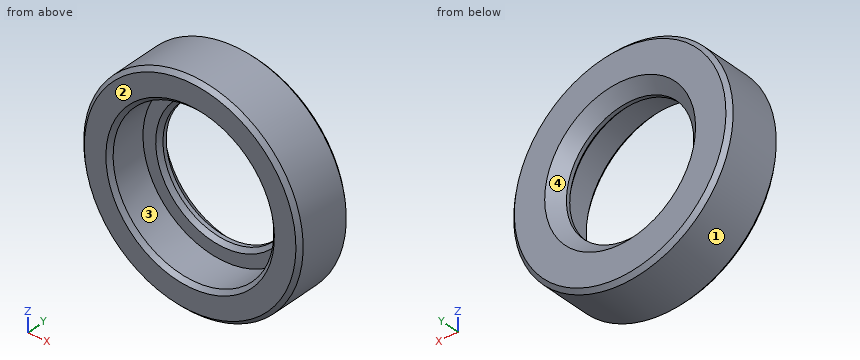
```python
from build123d import *

# Parameters (mm, degrees)
FASE1_SIZE = 0.2
FASE2_SIZE = 0.6


with BuildPart() as part:
    # Skizze1 → Rotation1 (revolve)
    with BuildSketch(Plane(origin=(0, 0, 0), x_dir=(0, 0, -1), z_dir=(1, 0, 0))):
        Polygon((4.1, -1.5), (4.1, 0.5), (3.25, 0.5), (3.25, 1.5), (5.6, 1.5), (5.6, -1.5), align=None)
    revolve(axis=Axis((0, 14.193037975, 0), (0, -1, 0)))

    # Fase1
    fase1_edges = [part.edges().sort_by_distance(p)[0] for p in [
        (0, -1.5, 5.6),
        (0, 1.5, 5.6),
        (0, 0.5, 3.25),
        (0, -1.5, 4.1),
    ]]
    chamfer(fase1_edges, length=FASE1_SIZE)

    # Fase2
    fase2_edges = [part.edges().sort_by_distance(p)[0] for p in [
        (0, 1.5, 3.25),
    ]]
    chamfer(fase2_edges, length=FASE2_SIZE)


solid = part.part
```
Could you check a few things on this model? Use its own coordinates, in mm. Face numbers are marked on the shaded views. Round coordinates to 2 decimals unless told otherwise and drop trailing zeros. Loops run counter-clockwise (first coordinate to the right, second up) from the corner with the lowest first, then second, coordinate; pieces in that order, holes last. Notation, with made-up numbers: (32, 84) - (84, 84) arc R17 ccw to (84, 102) - close; hole circle Ø4 at (12, -20.5). An arc over 180 degrees is marked (long way). Answer in a Markdown table with one row per item. Add a question column.
(1) If we section it at B-B (z = 0): Please give me the cut outline in (x, y).
(2) I'm going to push flat-ended pins straight in: pin 1 (1 mm diameter, centred on x = 1, z = 2.5, fed in from +Y); pin 2 (1.5 mm diameter, centred on y = -0.5, z = -2, fed in from +X); pin 3 (1.5 mm diameter, centred on x = 2.5, z = 1.5, fed in from +Y). Where does each tip first touch, or does it pass through?
(3) If we mould it in two halves opening along Z, with no side actions, what happens to the marked faces 1, 2, 3 and 4? For each: pulls with the +Z half, pulls with the -Z half, needs draft (parallel to the pull), parting line crosses it, or undercut.
(4) I need wall thicknesses on line 1 along X through (y, z) = (-0.05, 0); line 2 along X through (y, z) = (0.8, 0); line 3 along Y through (x, z) = (1.75, 3.5). Which ranges of each line are inside material? Lowest first, please.
(5) If we section it at D-D (y = 1.05): Please give me the cut outline in (x, z).
(6) If we section it at A-A (x = 0): Please give me the cut outline in (y, z).
(7) If we section it at C-C (y = -0.5): Please give me the cut outline in (x, z), plus the area to 3 significant figures.
Model answer:
| question | item | result |
|---|---|---|
| 1 | outline | (-5.6, -1.3) - (-5.4, -1.5) - (-4.3, -1.5) - (-4.1, -1.3) - (-4.1, 0.5) - (-3.45, 0.5) - (-3.25, 0.7) - (-3.25, 0.9) - (-3.85, 1.5) - (-5.4, 1.5) - (-5.6, 1.3) - close; (3.25, 0.7) - (3.45, 0.5) - (4.1, 0.5) - (4.1, -1.3) - (4.3, -1.5) - (5.4, -1.5) - (5.6, -1.3) - (5.6, 1.3) - (5.4, 1.5) - (3.85, 1.5) - (3.25, 0.9) - close |
| 2 | pin 1 | passes through |
| 2 | pin 2 | stops at x = 5.46 |
| 2 | pin 3 | stops at y = 1.32 |
| 3 | face 1 | parting line crosses it |
| 3 | face 2 | needs draft |
| 3 | face 3 | undercut |
| 3 | face 4 | undercut |
| 4 | line 1 | x = -5.6 to -4.1, 4.1 to 5.6 |
| 4 | line 2 | x = -5.6 to -3.25, 3.25 to 5.6 |
| 4 | line 3 | y = 0.5 to 1.5 |
| 5 | outline | circle Ø11.2 at (0, 0); hole circle Ø6.8 at (0, 0) |
| 6 | outline | (-1.5, -5.4) - (-1.3, -5.6) - (1.3, -5.6) - (1.5, -5.4) - (1.5, -3.85) - (0.9, -3.25) - (0.7, -3.25) - (0.5, -3.45) - (0.5, -4.1) - (-1.3, -4.1) - (-1.5, -4.3) - close; (-1.5, 4.3) - (-1.3, 4.1) - (0.5, 4.1) - (0.5, 3.45) - (0.7, 3.25) - (0.9, 3.25) - (1.5, 3.85) - (1.5, 5.4) - (1.3, 5.6) - (-1.3, 5.6) - (-1.5, 5.4) - close |
| 7 | outline | circle Ø11.2 at (0, 0); hole circle Ø8.2 at (0, 0) |
| 7 | area | 45.7 mm² |
